Drawing for the job (mm, zero at the part's lowest x, y, z). A direction names the side the tool comes from. Round coordinates to 2 decimals unless told otherwise and drop trailing zeros. Order: outer loops, then holes, each group sorted by start corner. A loop starts at its lowest first (then second) coordinate and runs counter-clockwise, first axis right, second up. Notation, with made-up numbers: (80.25, -8) -> (106.25, -8) arc R9 cw to (106.25, 8) -> close; hole circle Ø5 at (-39.5, 36.25). An arc over 180 degrees is marked (long way). Use CSV: the item, a comma, the result in double quotes.
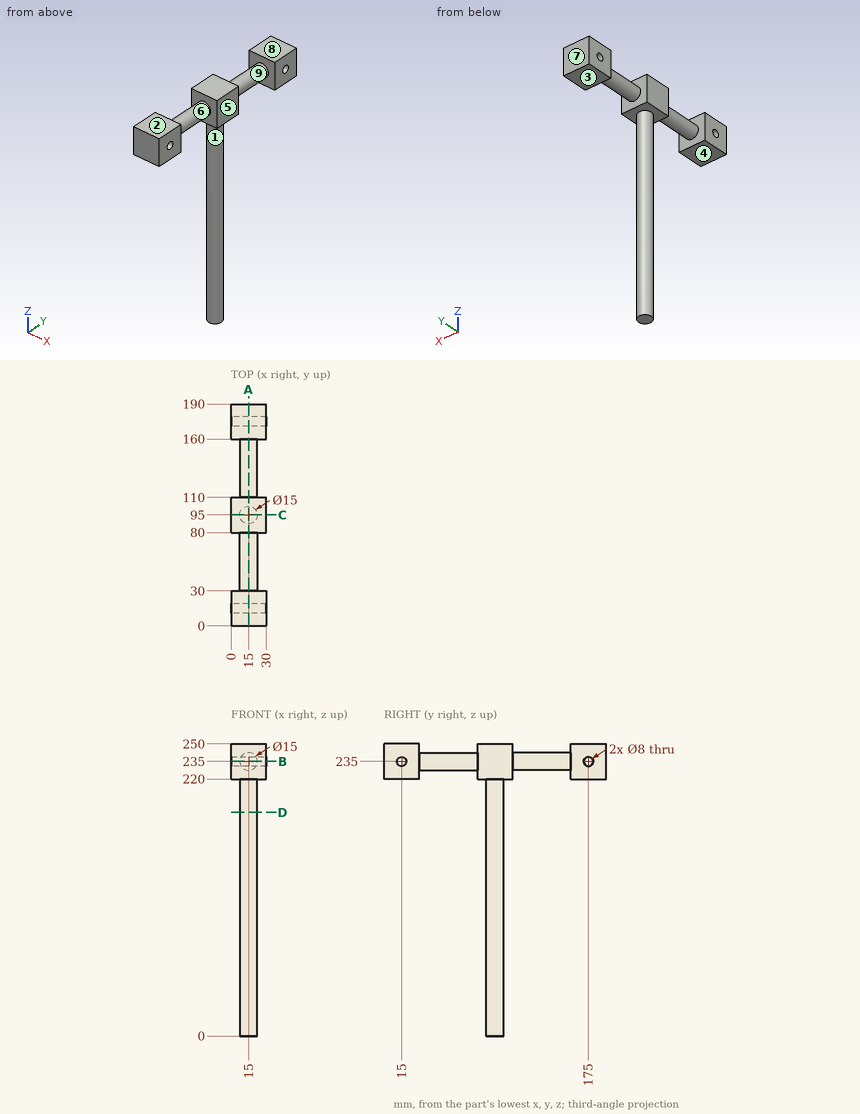
Q1. Which spindle directions (+Z, -Z, +X, -X, +Y, -Y) get a long thin tool onto all of the face, cutting with end or side? Do the marked faces 1, 2, 3, 4 and 5. Say none if no direction does.
From the geometry:
face 1,"-Z"
face 2,"+Z, +X, -X, +Y, -Y"
face 3,"-Z, +X, -X, +Y"
face 4,"-Z, +X, -X, -Y"
face 5,"+Z, -Z, +X, +Y, -Y"
Q2. Cut at D-D (z = 191.5). Give the cut face in (x, y).
From the geometry:
outline,"circle Ø15 at (15, 95)"
Q3. Mould opens along Y. For the marked faces 6, 7, 8 and 9 say: +Y half, -Y half, draft (parallel to the pull), parting line (faces both ways), or undercut.
From the geometry:
face 6,"undercut"
face 7,"+Y half"
face 8,"draft"
face 9,"undercut"
Q4. Cut at C-C (y = 95). Give the cut face in (x, z), plus the area to 3 significant figures.
From the geometry:
outline,"(0, 220) -> (7.5, 220) -> (7.5, 0) -> (22.5, 0) -> (22.5, 220) -> (30, 220) -> (30, 250) -> (0, 250) -> close"
area,"4,200 mm²"
Q5. Probe line 1 along Y through (x, z) = (21, 235); line 2 along Y through (x, z) = (26, 222); line 3 along Z through (x, y) = (21, 175). List the from-to ranges inside material, lowest first.
From the geometry:
line 1,"y = 0 to 11, 19 to 171, 179 to 190"
line 2,"y = 0 to 30, 80 to 110, 160 to 190"
line 3,"z = 220 to 231, 239 to 250"
Q6. Cut at A-A (x = 15). Give the cut face in (y, z), plus the area to 3 significant figures.
From the geometry:
outline,"(0, 220) -> (30, 220) -> (30, 227.5) -> (80, 227.5) -> (80, 220) -> (87.5, 220) -> (87.5, 0) -> (102.5, 0) -> (102.5, 220) -> (110, 220) -> (110, 227.5) -> (160, 227.5) -> (160, 220) -> (190, 220) -> (190, 250) -> (160, 250) -> (160, 242.5) -> (110, 242.5) -> (110, 250) -> (80, 250) -> (80, 242.5) -> (30, 242.5) -> (30, 250) -> (0, 250) -> close; hole circle Ø8 at (15, 235); hole circle Ø8 at (175, 235)"
area,"7,400 mm²"
Q7. Pin check, flat tips, straight feed: pin 1 (12 mm diameter, centred on x = 17, y = 65, fed in from -Z); pin 2 (4 mm diameter, centred on x = 9, z = 96.5, fed in from +Y); pin 3 (1.5 mm diameter, centred on x = 16.5, z = 209.5, fed in from +Y); pin 4 (9 mm diameter, centred on x = 17, z = 238, fed in from -Y). Stop position of each tip, or through.
From the geometry:
pin 1,"stops at z = 227.5"
pin 2,"stops at y = 101.34"
pin 3,"stops at y = 102.46"
pin 4,"stops at y = 0"
Q8. Cut at B-B (z = 235). Give the cut face in (x, y).
From the geometry:
outline,"(0, 0) -> (30, 0) -> (30, 11) -> (0, 11) -> close; (0, 19) -> (30, 19) -> (30, 30) -> (22.5, 30) -> (22.5, 80) -> (30, 80) -> (30, 110) -> (22.5, 110) -> (22.5, 160) -> (30, 160) -> (30, 171) -> (0, 171) -> (0, 160) -> (7.5, 160) -> (7.5, 110) -> (0, 110) -> (0, 80) -> (7.5, 80) -> (7.5, 30) -> (0, 30) -> close; (0, 179) -> (30, 179) -> (30, 190) -> (0, 190) -> close"
